Verification items for this drawing (mm, ordinates from the low corner). Give positions to 0.01 mm unless a question says otherwise; leave off trailing zeros. Order: outer loops, then holes, each group sorted by start corner. A loop starts at its lowest first (then second) coordinate and runs counter-clockwise, first axis right, second up. Notation, with made-up numbers: M 27.5,-20.75 L 86.5,-20.75 A18 cw 86.5,0.25 Z; hole C -32.75,49.5 d7. An arc over 180 degrees is marked long. Return JSON: item names as keys, results as strings. Group by question number.
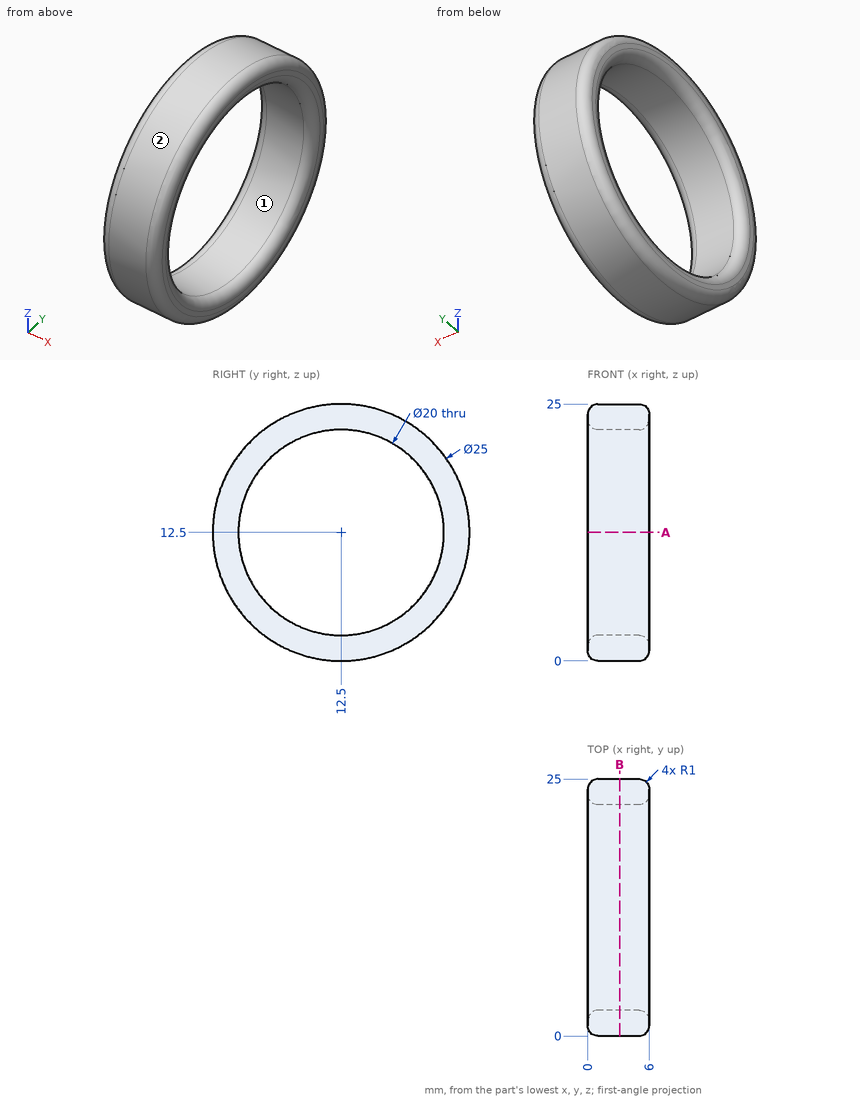
1) Material ranges on line 1 along Z through (x, y) = (4.15, 12.5); line 2 along Z through (x, y) = (2.2, 14.25); line 3 along Y through (x, z) = (4.05, 10), recorded low to high.
2) Sectioned sample at B-B on x = 3.1. Record the boundary of the cut face in (y, z), then the cut area to 3 significant figures.
3) Sectioned sample at A-A on z = 12.5. Record the boundary of the cut face in (x, y), then the cut area to 3 significant figures.
4) Release check for a two-part mould opening along Z. For the marked faces 1 and 2 record: released by +Z, released by -Z, zero draft, split by the parting line, or undercut.
5) Depth check by flat-ended pin: P1, Ø1, axis at x = 4.5, y = 9.5, coming from the +Z side. Enter the tip coordinate at first touch or a pass-through.
Reply:
{
 "1": {"line 1": "0 to 2.5, 22.5 to 25", "line 2": "0.12 to 2.65, 22.35 to 24.88", "line 3": "0.25 to 2.82, 22.18 to 24.75"},
 "2": {"outline": "C 12.5,12.5 d25; hole C 12.5,12.5 d20", "area": "177 mm^2"},
 "3": {"outline": "M 0,1 A1 ccw 1,0 L 5,0 A1 ccw 6,1 L 6,1.5 A1 ccw 5,2.5 L 1,2.5 A1 ccw 0,1.5 Z; M 0,23.5 A1 ccw 1,22.5 L 5,22.5 A1 ccw 6,23.5 L 6,24 A1 ccw 5,25 L 1,25 A1 ccw 0,24 Z", "area": "28.3 mm^2"},
 "4": {"face 1": "undercut", "face 2": "split by the parting line"},
 "5": {"P1": "z = 24.75"}
}
